from build123d import *

# Parameters (mm, degrees)
CROQUIS1_W              = 32
CROQUIS1_H              = 45
CROQUIS1_R              = 5
SALIENTE_EXTRUIR1_DEPTH = 3
CROQUIS2_W              = 32
CROQUIS2_H              = 3
SALIENTE_EXTRUIR2_DEPTH = 80
REDONDEO1_R             = 3
REDONDEO3_R             = 1
CROQUIS5_R              = 1.75
CORTAR_EXTRUIR2_DEPTH   = 10
CROQUIS6_R              = 1.75
CORTAR_EXTRUIR3_DEPTH   = 10
REDONDEO4_R             = 10
CROQUIS7_R              = 2
CORTAR_EXTRUIR4_DEPTH   = 10


with BuildPart() as part:
    # Croquis1 → Saliente-Extruir1 (new body)
    with BuildSketch(Plane(origin=(0, 0, 0), x_dir=(1, 0, 0), z_dir=(0, 1, 0))):
        Rectangle(CROQUIS1_W, CROQUIS1_H)
        with Locations(Location((0, 12.5, 0), (0, 0, 270))):
            Circle(CROQUIS1_R, mode=Mode.SUBTRACT)
    extrude(amount=SALIENTE_EXTRUIR1_DEPTH)

    # Croquis2 → Saliente-Extruir2 (add)
    with BuildSketch(Plane.XZ):
        with Locations((0, 21)):
            Rectangle(CROQUIS2_W, CROQUIS2_H)
    extrude(amount=SALIENTE_EXTRUIR2_DEPTH)

    # Redondeo1
    redondeo1_edges = [part.edges().sort_by_distance(p)[0] for p in [
        (0, 0, 19.5),
    ]]
    fillet(redondeo1_edges, radius=REDONDEO1_R)

    # Redondeo3
    redondeo3_edges = [part.edges().sort_by_distance(p)[0] for p in [
        (-16, 3, 0),
        (16, 3, 0),
    ]]
    fillet(redondeo3_edges, radius=REDONDEO3_R)

    # Croquis5 → Cortar-Extruir2 (cut)
    with BuildSketch(Plane(origin=(0, 3, 0), x_dir=(1, 0, 0), z_dir=(0, 1, 0))):
        with Locations(Location((-8.25, 12.5, 0), (0, 0, 270))):
            Circle(CROQUIS5_R)
        with Locations(Location((8.25, 12.5, 0), (0, 0, 270))):
            Circle(CROQUIS5_R)
    extrude(amount=-CORTAR_EXTRUIR2_DEPTH, mode=Mode.SUBTRACT)

    # Croquis6 → Cortar-Extruir3 (cut)
    with BuildSketch(Plane.XY.offset(22.5)):
        with Locations((-9, -63)):
            Circle(CROQUIS6_R)
        with Locations((9, -63)):
            Circle(CROQUIS6_R)
    extrude(amount=-CORTAR_EXTRUIR3_DEPTH, mode=Mode.SUBTRACT)

    # Redondeo4
    redondeo4_edges = [part.edges().sort_by_distance(p)[0] for p in [
        (-16, -80, 21),
        (16, -80, 21),
    ]]
    fillet(redondeo4_edges, radius=REDONDEO4_R)

    # Croquis7 → Cortar-Extruir4 (cut)
    with BuildSketch(Plane(origin=(0, 3, 0), x_dir=(1, 0, 0), z_dir=(0, 1, 0))):
        with Locations(Location((0, -2.5, 0), (0, 0, 270))):
            Circle(CROQUIS7_R)
    extrude(amount=-CORTAR_EXTRUIR4_DEPTH, mode=Mode.SUBTRACT)


solid = part.part
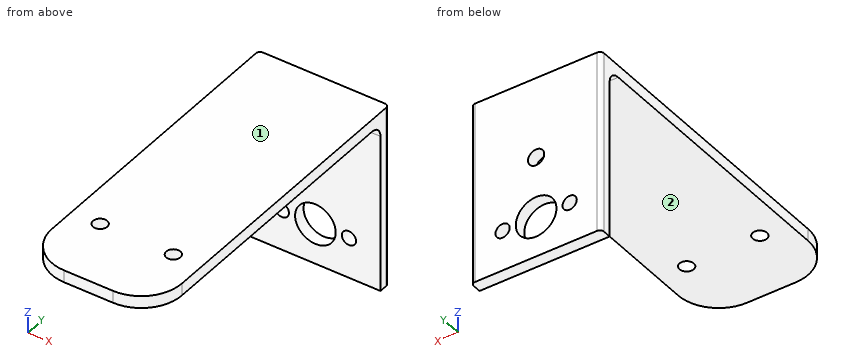
Could you check a few things on this model? Use its own coordinates, in mm. Face numbers are marked on the shaded views. A direction names the side the tool comes from. Round coordinates to 2 decimals unless told otherwise and drop trailing zeros. Order: outer loops, then holes, each group sorted by start corner. A loop starts at its lowest first (then second) coordinate and runs counter-clockwise, first axis right, second up. Notation, with made-up numbers: M 17,26 L 67,26 A26 ccw 67,47 Z; hole C -13,-7 d8. An arc over 180 degrees is marked long. One line per item, written item: value.
(1) Imagine slicing it at B-B (y = -63). Write out the boundary of the cut face in (x, z).
Ans:
outline: M -16,19.5 L -10.75,19.5 L -10.75,22.5 L -16,22.5 Z; M -7.25,19.5 L 7.25,19.5 L 7.25,22.5 L -7.25,22.5 Z; M 10.75,19.5 L 16,19.5 L 16,22.5 L 10.75,22.5 Z
(2) Imagine slicing it at C-C (z = 2.5). Write out the boundary of the cut face in (x, y).
Ans:
outline: M -16,0 L -2,0 L -2,3 L -15,3 A1 ccw -16,2 Z; M 2,0 L 16,0 L 16,2 A1 ccw 15,3 L 2,3 Z
(3) I'm going to push flat-ended pins straight in: P1, Ø2.5, axis at x = 0, z = 2.5, coming from the +Y side; P2, Ø4.5, axis at x = -8.25, z = -12.5, coming from the +Y side; P3, Ø16, axis at x = 0, z = -12.5, coming from the -Y side; P4, Ø8, axis at x = 10, y = -53.5, coming from the -Z side. Where does each tip first touch, or does it pass through?
Ans:
P1: passes through
P2: stops at y = 3
P3: stops at y = 0
P4: stops at z = 19.5
(4) Imagine slicing it at A-A (z = -12.5). Write out the boundary of the cut face in (x, y), and give its area (3 significant figures).
Ans:
outline: M -16,0 L -10,0 L -10,3 L -15,3 A1 ccw -16,2 Z; M -6.5,0 L -5,0 L -5,3 L -6.5,3 Z; M 5,0 L 6.5,0 L 6.5,3 L 5,3 Z; M 10,0 L 16,0 L 16,2 A1 ccw 15,3 L 10,3 Z
area: 44.6 mm^2
(5) Imagine slicing it at D-D (x = 8.25). Write out the boundary of the cut face in (y, z).
Ans:
outline: M -79.74,19.5 L -64.58,19.5 L -64.58,22.5 L -79.74,22.5 Z; M -61.42,19.5 L -3,19.5 A3 cw 0,16.5 L 0,-10.75 L 3,-10.75 L 3,22.5 L -61.42,22.5 Z; M 0,-22.5 L 3,-22.5 L 3,-14.25 L 0,-14.25 Z
(6) I need wall thicknesses on line 1 along X through (y, z) = (2, -12.5); line 2 along Z through (x, y) = (8, 1); line 3 along Y through (x, z) = (-11, -13). Which ranges of each line are inside material? Lowest first, please. Write a range as from..to.
Ans:
line 1: x = -16..-10, -6.5..-5, 5..6.5, 10..16
line 2: z = -22.5..-14.23, -10.77..22.5
line 3: y = 0..3
(7) Which directions (+Z, -Z, +X, -X, +Y, -Y) give clear straight access to the entire face, cutting with the end or side of a thin tool? Please do the marked faces 1 and 2.
Ans:
face 1: +Z, +X, -X, +Y, -Y
face 2: -Z, +X, -X, -Y
